from build123d import *

# Parameters (mm, degrees)
BOSS_EXTRUDE1_DEPTH = 30
BOSS_EXTRUDE3_DEPTH = 30
LPATTERN1_COUNT     = 35
LPATTERN1_PITCH     = 2


with BuildPart() as part:
    # Sketch2 → Boss-Extrude1 (new body)
    with BuildSketch(Plane.XY):
        Polygon((-35, 30), (-20, 70), (0, 70), (0, 0), (-35, 0), align=None)
    extrude(amount=BOSS_EXTRUDE1_DEPTH)

    # Sketch3 → Boss-Extrude3 (add)
    with BuildSketch(Plane.XY.offset(30)):
        Polygon((0, 70), (2, 69), (0, 68), align=None)
    boss_extrude3 = extrude(amount=-BOSS_EXTRUDE3_DEPTH)

    # LPattern1: Boss-Extrude3 ×35
    with Locations(*[(0, -i * LPATTERN1_PITCH, 0) for i in range(1, LPATTERN1_COUNT)]):
        add(boss_extrude3)


solid = part.part
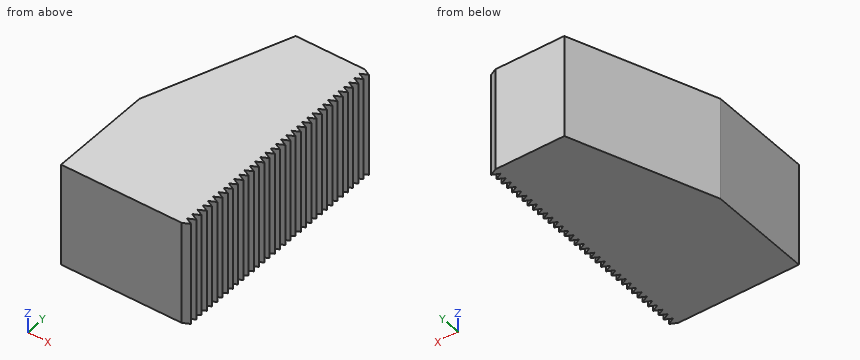
Work out the finished part from the listing and answer in its coordinate system (mm). Give positions to 0.01 mm unless a question says otherwise; leave off trailing zeros. Order: outer loops, then holes, each group sorted by start corner. A loop starts at its lowest first (then second) coordinate and runs counter-clockwise, first axis right, second up. Notation, with made-up numbers: M -25.75,-23 L 26.25,-23 A25 cw 26.25,9 Z; hole C -30.5,-35.75 d6. An arc over 180 degrees is marked long. Return JSON: item names as keys, results as strings.
Q1. Find the intervals of material crossed by line 1 along X through (y, z) = (6.5, 11.75); line 2 along X through (y, z) = (67.5, 4.75), in increasing order. Write a range as [from, to].
Answer below:
{"line 1": "x = [-35, 1]", "line 2": "x = [-20.94, 1]"}
Q2. Find section A-A, the plane x = -22.5. Write down the section's boundary in (y, z).
Answer below:
{"outline": "M 0,0 L 63.33,0 L 63.33,30 L 0,30 Z"}
Q3. Each of these flat-tipped pins is pushed along its axis until it touches: pin 1 (8 mm diameter, centred on y = 52, z = 12, fed in from -X); pin 2 (6 mm diameter, centred on y = 22.5, z = 13.5, fed in from +X); pin 3 (1 mm diameter, centred on y = 16, z = 11.5, fed in from +X). Where does it stop, or does it pass through?
Answer below:
{"pin 1": "stops at x = -28.25", "pin 2": "stops at x = 2", "pin 3": "stops at x = 1"}
